Input: part model. Units: mm. Frame: model coordinates. Face numbers are marked on the shaded views. A direction names the side the tool comes from. Round coordinates to 2 decimals unless told otherwise and drop trailing zeros. Loops run counter-clockwise (first coordinate to the right, second up) from the corner with the lowest first, then second, coordinate; pieces in that order, holes last. Notation, with made-up numbers: M -0.5,-15.75 L 19.5,-15.75 A21 cw 19.5,-1.75 Z; hole C -32.75,-33.5 d4. An arc over 180 degrees is marked long. Return JSON: item names as keys, results as strings. Group by question number.
1) Section B-B (z = 0). Output: boundary loops of the cut face in (x, y).
2) Section C-C (z = 5.75). Output: boundary loops of the cut face in (x, y), plus the area to 3 significant figures.
3) Access query for the marked faces 1 and 2. Directions: +Z, -Z, +X, -X, +Y, -Y. A direction counts if a zero-diameter tool reaches every point of the face in a straight line with its end or side. Return the directions, or none.
4) Section D-D (x = 2). Output: boundary loops of the cut face in (y, z), plus the area to 3 significant figures.
5) Contact query for flat-ended pins moving along their axis: P1, Ø3, axis at x = 85.5, z = -3, coming from the -Y side; P2, Ø5, axis at x = 0, y = 0, coming from the -Z side; P3, Ø2, axis at y = 2, z = -4.5, coming from the -X side; P4, Ø3, axis at y = 4, z = -4, coming from the -X side. Output: stop coordinate, or through.
6) Section A-A (x = 88.5). Output: boundary loops of the cut face in (y, z), plus the area to 3 significant figures.
7) Material intervals for line 1 (X direction, y = 2.55, z = 0); line 2 (Y direction, x = 0, z = 6); line 3 (Z direction, x = 6, y = -1), sorted ascending. Write a range as from..to.
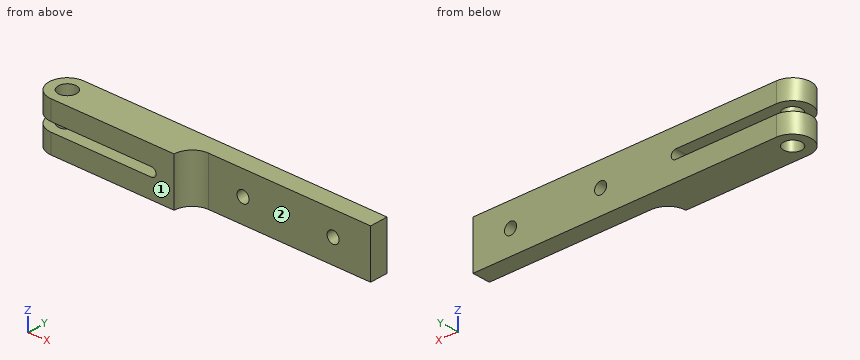
from build123d import *

# Parameters (mm, degrees)
SKETCH2_R           = 3
BOSS_EXTRUDE1_DEPTH = 8
SKETCH3_R           = 2
CUT_EXTRUDE1_DEPTH  = 103.02450686


with BuildPart() as part:
    # Sketch2 → Boss-Extrude1 (new, symmetric)
    with BuildSketch(Plane.XY):
        with BuildLine():
            Line((0, -6), (41, -6))
            ThreePointArc((41, -6), (42.757359313, -1.757359313), (47, 0))
            Line((47, 0), (101, 0))
            Line((101, 0), (101, 6))
            Line((101, 6), (0, 6))
            ThreePointArc((0, 6), (-6, 0), (0, -6))
        make_face()
        Circle(SKETCH2_R, mode=Mode.SUBTRACT)
    extrude(amount=BOSS_EXTRUDE1_DEPTH, both=True)

    # Sketch3 → Cut-Extrude1 (cut, through all)
    with BuildSketch(Plane(origin=(0, 6, 0), x_dir=(1, 0, 0), z_dir=(0, 1, 0))):
        with Locations(Location((58.5, 0, 0), (0, 0, 270))):
            Circle(SKETCH3_R)
        with Locations(Location((88.5, 0, 0), (0, 0, 270))):
            Circle(SKETCH3_R)
        with BuildLine():
            Line((33.49999953, -1.5), (-6, -1.5))
            Line((-6, -1.5), (-6, 1.5))
            Line((-6, 1.5), (33.49999953, 1.5))
            ThreePointArc((33.49999953, 1.5), (35, 0), (33.49999953, -1.5))
        make_face()
    extrude(amount=-CUT_EXTRUDE1_DEPTH, mode=Mode.SUBTRACT)


solid = part.part
Returned:
{
 "1": {"outline": "M 35,-6 L 41,-6 A6 cw 47,0 L 56.5,0 L 56.5,6 L 35,6 Z; M 60.5,0 L 86.5,0 L 86.5,6 L 60.5,6 Z; M 90.5,0 L 101,0 L 101,6 L 90.5,6 Z"},
 "2": {"outline": "M 0,-6 L 41,-6 A6 cw 47,0 L 101,0 L 101,6 L 0,6 A6 ccw Z; hole C 0,0 d6", "area": "888 mm^2"},
 "3": {"face 1": "+Z, -Z, +X, -X, -Y", "face 2": "+Z, -Z, +X, -Y"},
 "4": {"outline": "M -6,-8 L -2.24,-8 L -2.24,-1.5 L -6,-1.5 Z; M -6,1.5 L -2.24,1.5 L -2.24,8 L -6,8 Z; M 2.24,-8 L 6,-8 L 6,-1.5 L 2.24,-1.5 Z; M 2.24,1.5 L 6,1.5 L 6,8 L 2.24,8 Z", "area": "97.9 mm^2"},
 "5": {"P1": "stops at y = 0", "P2": "passes through", "P3": "stops at x = -5.92", "P4": "stops at x = -5.45"},
 "6": {"outline": "M 0,-8 L 6,-8 L 6,-2 L 0,-2 Z; M 0,2 L 6,2 L 6,8 L 0,8 Z", "area": "72.0 mm^2"},
 "7": {"line 1": "x = 35..56.5, 60.5..86.5, 90.5..101", "line 2": "y = -6..-3, 3..6", "line 3": "z = -8..-1.5, 1.5..8"}
}
